from build123d import *

# Parameters (mm, degrees)
SKETCH1_W           = 40
SKETCH1_H           = 30
BOSS_EXTRUDE1_DEPTH = 12
SKETCH2_W           = 25
SKETCH2_H           = 12
CUT_EXTRUDE1_DEPTH  = 12
SKETCH3_R           = 4
CUT_EXTRUDE2_DEPTH  = 100
FILLET1_R           = 5
SKETCH4_R           = 4
CUT_EXTRUDE3_DEPTH  = 12.5
CHAMFER1_SIZE       = 2


with BuildPart() as part:
    # Sketch1 → Boss-Extrude1 (new body)
    with BuildSketch(Plane(origin=(0, 0, 0), x_dir=(1, 0, 0), z_dir=(0, 1, 0))):
        Rectangle(SKETCH1_W, SKETCH1_H)
    extrude(amount=BOSS_EXTRUDE1_DEPTH)

    # Sketch2 → Cut-Extrude1 (cut)
    with BuildSketch(Plane(origin=(0, 12, 0), x_dir=(1, 0, 0), z_dir=(0, 1, 0))):
        with Locations((0, 9)):
            Rectangle(SKETCH2_W, SKETCH2_H)
    extrude(amount=-CUT_EXTRUDE1_DEPTH, mode=Mode.SUBTRACT)

    # Sketch3 → Cut-Extrude2 (cut)
    with BuildSketch(Plane(origin=(20, 0, 0), x_dir=(0, 0, -1), z_dir=(1, 0, 0))):
        with Locations((9, 6)):
            Circle(SKETCH3_R)
    extrude(amount=-CUT_EXTRUDE2_DEPTH, mode=Mode.SUBTRACT)

    # Fillet1
    fillet1_edges = [part.edges().sort_by_distance(p)[0] for p in [
        (-16.25, 0, -15),
        (-16.25, 12, -15),
        (16.25, 0, -15),
        (16.25, 12, -15),
    ]]
    fillet(fillet1_edges, radius=FILLET1_R)

    # Sketch4 → Cut-Extrude3 (cut)
    with BuildSketch(Plane.XY.offset(15)):
        with Locations((-12.5, 6)):
            Circle(SKETCH4_R)
        with Locations((12.5, 6)):
            Circle(SKETCH4_R)
    extrude(amount=-CUT_EXTRUDE3_DEPTH, mode=Mode.SUBTRACT)

    # Chamfer1
    chamfer1_edges = [part.edges().sort_by_distance(p)[0] for p in [
        (0, 12, 15),
        (12.5, 0, -6.5),
        (12.5, 12, -6.5),
        (0, 12, -3),
        (-12.5, 6, -15),
        (-20, 6, -15),
        (20, 12, 2.5),
        (-20, 0, 2.5),
        (-20, 12, 2.5),
        (-20, 10.535533906, -13.535533906),
        (-20, 1.464466094, -13.535533906),
        (-12.5, 0, -6.5),
        (-12.5, 12, -6.5),
        (-12.5, 10.535533906, -13.535533906),
        (-12.5, 1.464466094, -13.535533906),
        (12.5, 6, -15),
        (20, 6, -15),
        (12.5, 10.535533906, -13.535533906),
        (12.5, 1.464466094, -13.535533906),
        (20, 10.535533906, -13.535533906),
        (20, 1.464466094, -13.535533906),
        (20, 0, 2.5),
    ]]
    chamfer(chamfer1_edges, length=CHAMFER1_SIZE - 0.0001)  # a hair under: the kernel refuses the full size


solid = part.part
Design review of the part built by this model. Coordinates are the model's own, in mm. A direction names the side the tool comes from. Round coordinates to 2 decimals unless told otherwise and drop trailing zeros. Write each loop counter-clockwise with the first axis right and the second up, starting at its lowest first coordinate (ties: lowest second). Pieces come first, ordered by that corner, then holes. Notation, with made-up numbers: (75, 70.25) -> (85, 70.25) arc R17 cw to (85, 89.25) -> close; hole circle Ø2 at (58, 51.25). An arc over 180 degrees is marked (long way). One line per question, with ' | ' between items.
(1) Insertion check: P1, Ø3, axis at x = 3.5, y = 3, coming from the -Z side; P2, Ø7, axis at x = -12.5, y = 6, coming from the -Z side; P3, Ø2.5, axis at x = -12.5, y = 5.5, coming from the +Z side. Each pin has a flat end and moves straight along its axis. Give the tip position at first contact, or say it passes through.
Result sheet:
P1: z = -3 | P2: z = -15 | P3: z = 2.5
(2) Take a section at D-D, the plane z = -3.5. State the section outline as (x, y) points.
Result sheet:
outline: (-20, 2) -> (-18, 0) -> (-14.5, 0) -> (-12.5, 2) -> (-12.5, 10) -> (-14.5, 12) -> (-18, 12) -> (-20, 10) -> close; (12.5, 2) -> (14.5, 0) -> (18, 0) -> (20, 2) -> (20, 10) -> (18, 12) -> (14.5, 12) -> (12.5, 10) -> close
(3) Draft analysis for pull direction X (two halves, no side actions). For faces 1 (the conical face through (19.24, 2.37, -12.69)), 2 (the flat face through (0, 11, -2)), 3 (the flat face through (-19, 1, 3)), 4 (the flat face through (-13.5, 11, -6.4)), state which applies: released by +X, released by -X, zero draft, split by the parting line, or undercut.
Result sheet:
face 1: released by +X | face 2: undercut | face 3: released by -X | face 4: undercut
(4) Wall thickness on line 1 (X direction, y = 7, z = 3.5); line 2 (Y direction, x = -12.5, z = 9.5); line 3 (Z direction, x = 9.5, y = 9.75): over which ranges is each line inside the solid? List them lowest first. Write a range as [from, to].
Result sheet:
line 1: [-20, -16.37], [-8.63, 8.63], [16.37, 20] | line 2: [0, 2], [10, 12] | line 3: [-3, 15]
(5) Machinability: for faces 5 (the conical face through (13.26, 2.31, -12.63)), 6 (the flat face through (12.5, 6.3, -4.6)), 7 (the flat face through (-19, 11, 2)), 8 (the conical face through (13.26, 9.63, -12.69)), 9 (the flat face through (0, 11, 14)), which of the approach directions +Z, -Z, +X, -X, +Y, -Y give a long, thin tool a straight path to every point of the face, cutting with its end or side? Answer none if there is none.
Result sheet:
face 5: -Z, -Y | face 6: -Z, +Y, -Y | face 7: +Z, -Z, -X, +Y | face 8: -Z, +Y | face 9: +Z, +X, -X, +Y
(6) Take a section at A-A, the plane z = -9. State how many separate pieces and enclosed holes the cut face has, and give its area (3 significant figures).
Result sheet:
separate pieces: 4 | enclosed holes: 0 | area: 44.0 mm2
(7) Take a section at C-C, the plane x = -17. State the section outline as (y, z) points.
Result sheet:
outline: (0, -10) arc R5 ccw to (5, -15) -> (7, -15) arc R5 ccw to (12, -10) -> (12, 13) -> (10, 15) -> (0, 15) -> close; hole circle Ø8 at (6, -9)
